```python
from build123d import *

# Parameters (mm, degrees)
SKETCH1_W                = 31
SKETCH1_H                = 7
SKETCH1_W_2              = 100
SKETCH1_H_2              = 45
BOSS_EXTRUDE1_DEPTH      = 7
F_6_0_6_DIAMETER_HOLE1_D = 6


with BuildPart() as part:
    # Sketch1 → Boss-Extrude1 (new body)
    with BuildSketch(Plane(origin=(0, 0, 0), x_dir=(1, 0, 0), z_dir=(0, 1, 0))):
        with BuildLine():
            Line((-31, 0), (0, 0))
            Line((0, 0), (0, 4.7))
            ThreePointArc((0, 4.7), (-8, 12.7), (0, 20.7))
            Line((0, 20.7), (0, 84.468576745))
            Line((0, 84.468576745), (-100, 84.468576745))
            Line((-100, 84.468576745), (-100, 25.4))
            Line((-100, 25.4), (-74.6, 25.4))
            Line((-74.6, 25.4), (-74.6, 0))
            Line((-74.6, 0), (-31, 0))
        make_face()
        with Locations((-15.5, -3.5)):
            Rectangle(SKETCH1_W, SKETCH1_H)
        with Locations((-50, 106.968576745)):
            Rectangle(SKETCH1_W_2, SKETCH1_H_2)
    boss_extrude1 = extrude(amount=BOSS_EXTRUDE1_DEPTH)

    # Mirror1: Boss-Extrude1 across Right Plane
    add(boss_extrude1.mirror(Plane(origin=(0, 0, 0), x_dir=(0, 0, -1), z_dir=(1, 0, 0))))

    # Ø6.0 (6) Diameter Hole1 (through all)
    with Locations(Plane(origin=(-37.75, 7, -7.5), x_dir=(0, 0, 1), z_dir=(0, 1, 0))):
        with Locations((0, 0), (0, 75.5), (-105, 75.5), (-105, 0)):
            Hole(F_6_0_6_DIAMETER_HOLE1_D / 2)


solid = part.part
```
Geometry check sheet. Reference: the model listing, model coordinates, mm. A direction names the side the tool comes from. Round coordinates to 2 decimals unless told otherwise and drop trailing zeros. Order: outer loops, then holes, each group sorted by start corner. A loop starts at its lowest first (then second) coordinate and runs counter-clockwise, first axis right, second up. Notation, with made-up numbers: (43.25, 34) - (60.25, 34) arc R22 ccw to (60.25, 54) - close; hole circle Ø2 at (50.5, 42.25). An arc over 180 degrees is marked (long way). Use a Markdown table: item, result. Add a question column.
(1) Release check for a two-part mould opening along X. For faces 4 (the flat face through (1, 0, -62)), 5 (the cylindrical face through (-36.85, 3.45, -115.36)), 6 (the flat face through (74.6, 3, -13)), 7 (the cylindrical face through (-35.22, 3.45, -9.11)) record: pulls with the +X half, pulls with the -X half, needs draft (parallel to the pull), parting line crosses it, or undercut.
(2) Material ranges on line 1 along X through (y, z) = (4.75, -112.5); line 2 along X through (y, z) = (2.25, -12.7); line 3 along X through (y, z) = (2, -7.5), recorded low to high. Write a range as [from, to].
(3) Sectioned sample at B-B, the plane z = -112.5. Enter the section's corners in (x, y), and give its area (3 significant figures).
(4) Sectioned sample at D-D, the plane z = -12.7. Enter the section's corners in (x, y).
(5) Sectioned sample at A-A, the plane x = 0. Enter the section's corners in (y, z), and give its area (3 significant figures).
(6) Tool access check on faces 1 (the flat face through (-100, 3, -78)), 2 (the flat face through (-87, 3, -25.4)), 3 (the flat face through (53, 3, 0)). Record the directions out of +Z, -Z, +X, -X, +Y, -Y that give a thin tool (end or side, any length) a straight path to the whole face; none if there is none.
(7) Sectioned sample at C-C, the plane x = 37.75. Enter the section's corners in (y, z).
(8) Depth check by flat-ended pin: pin 1 (5.5 mm diameter, centred on x = 37.75, z = -112.5, fed in from -Y); pin 2 (3.5 mm diameter, centred on x = 84, y = 2, fed in from +Z); pin 3 (3.5 mm diameter, centred on x = -44.5, y = 4.5, fed in from +Z); pin 4 (3.5 mm diameter, centred on y = 2, z = -8, fed in from -X). Enter the tip coordinate at first touch or a pass-through.
Answers below:
| question | item | result |
|---|---|---|
| 1 | face 4 | needs draft |
| 1 | face 5 | undercut |
| 1 | face 6 | pulls with the +X half |
| 1 | face 7 | undercut |
| 2 | line 1 | [-100, -40.75], [-34.75, 34.75], [40.75, 100] |
| 2 | line 2 | [-74.6, -8], [8, 74.6] |
| 2 | line 3 | [-74.6, -40.75], [-34.75, -6.08], [6.08, 34.75], [40.75, 74.6] |
| 3 | outline | (-100, 0) - (-40.75, 0) - (-40.75, 7) - (-100, 7) - close; (-34.75, 0) - (34.75, 0) - (34.75, 7) - (-34.75, 7) - close; (40.75, 0) - (100, 0) - (100, 7) - (40.75, 7) - close |
| 3 | area | 1,320 mm² |
| 4 | outline | (-74.6, 0) - (-8, 0) - (-8, 7) - (-74.6, 7) - close; (8, 0) - (74.6, 0) - (74.6, 7) - (8, 7) - close |
| 5 | outline | (0, -129.47) - (7, -129.47) - (7, -20.7) - (0, -20.7) - close; (0, -4.7) - (7, -4.7) - (7, 7) - (0, 7) - close |
| 5 | area | 843 mm² |
| 6 | face 1 | +Z, -Z, -X, +Y, -Y |
| 6 | face 2 | +Z, -X, +Y, -Y |
| 6 | face 3 | +Z, +X, +Y, -Y |
| 7 | outline | (0, -129.47) - (7, -129.47) - (7, -115.5) - (0, -115.5) - close; (0, -109.5) - (7, -109.5) - (7, -10.5) - (0, -10.5) - close; (0, -4.5) - (7, -4.5) - (7, 0) - (0, 0) - close |
| 8 | pin 1 | through |
| 8 | pin 2 | z = -25.4 |
| 8 | pin 3 | z = 0 |
| 8 | pin 4 | x = -74.6 |
